Input: part model. Units: mm. Frame: model coordinates. A direction names the side the tool comes from. Coordinates: 2 decimals unless noted, no trailing zeros. Order: outer loops, then holes, each group sorted by start corner. A loop starts at its lowest first (then second) coordinate and runs counter-clockwise, first axis right, second up. Notation, with made-up numbers: (68.25, 48.5) -> (98.25, 48.5) arc R15 ccw to (98.25, 58.5) -> close; hole circle Ø10 at (50.5, -8.75). An arc over 180 degrees is marked (long way). Use CSV: the item, a comma, the result in double quotes. Start each with the question number.
```python
from build123d import *

# Parameters (mm, degrees)
BOSS_EXTRUDE1_DEPTH = 180
CUT_EXTRUDE1_REACH  = 186.932
SKETCH2_R           = 4
CUT_EXTRUDE2_REACH  = 186.932
SKETCH3_R           = 4


with BuildPart() as part:
    # Sketch1 → Boss-Extrude1 (new, symmetric)
    with BuildSketch(Plane.XY):
        Polygon((0, 0), (-30, 0), (-30, -2), (-2, -2), (-2, -30), (0, -30), align=None)
    extrude(amount=BOSS_EXTRUDE1_DEPTH, both=True)

    # Sketch2 → Cut-Extrude1 (cut, up to next)
    with BuildSketch(Plane(origin=(0, 0, 0), x_dir=(1, 0, 0), z_dir=(0, 1, 0)), mode=Mode.PRIVATE) as cut_extrude1_sk1:
        with Locations(Location((-15, 170, 0), (0, 0, 180))):
            Circle(SKETCH2_R)
    cut_extrude1_tool1 = extrude(cut_extrude1_sk1.sketch, amount=-CUT_EXTRUDE1_REACH, mode=Mode.PRIVATE) & part.part
    cut_extrude1 = cut_extrude1_tool1.solids().sort_by_distance((-15, 0, -170))[0]
    add(cut_extrude1, mode=Mode.SUBTRACT)

    # Sketch3 → Cut-Extrude2 (cut, up to next)
    with BuildSketch(Plane(origin=(0, 0, 0), x_dir=(0, 0, -1), z_dir=(1, 0, 0)), mode=Mode.PRIVATE) as cut_extrude2_sk1:
        with Locations(Location((157.5, -15, 0), (0, 0, 90))):
            Circle(SKETCH3_R)
    cut_extrude2_tool1 = extrude(cut_extrude2_sk1.sketch, amount=-CUT_EXTRUDE2_REACH, mode=Mode.PRIVATE) & part.part
    cut_extrude2 = cut_extrude2_tool1.solids().sort_by_distance((0, -15, -157.5))[0]
    add(cut_extrude2, mode=Mode.SUBTRACT)

    # Mirror1: Cut-Extrude1, Cut-Extrude2 across plane
    add(cut_extrude1.mirror(Plane.XY), mode=Mode.SUBTRACT)
    add(cut_extrude2.mirror(Plane.XY), mode=Mode.SUBTRACT)


solid = part.part
```
1. Section A-A on y = -15. Return loops of the section in (x, z).
2. Access query for faces 1 (the face through (-16, -2, 3)), 2 (the face through (-0.986, -15.521, -153.534)). Directions: +Z, -Z, +X, -X, +Y, -Y. A direction counts if a zero-diameter tool reaches every point of the face in a straight line with its end or side. Return the directions, or none.
3. Section B-B on z = 157.5. Return loops of the section in (x, y), then the cut area to 3 significant figures.
4. Material intervals for line 1 along Z through (x, y) = (-15, -1.15); line 2 along Z through (x, y) = (-1.4, -15); line 3 along Y through (x, z) = (-1.35, 157.5), sorted ascending.
5. Section D-D on z = -82.5. Return loops of the section in (x, y), then the cut area to 3 significant figures.
6. Pull-direction query (X, two-part tool) for faces 3 (the face through (-8.4, -1.6, -180)), 4 (the face through (0, -15, 3)), 5 (the face through (-14.479, -0.986, 166.034)); classes: released by +X, released by -X, zero draft, split by the parting line, or undercut.
7. Section C-C on x = -15. Return loops of the section in (y, z), then the cut area to 3 significant figures.
8. Contact query for flat-ended pins moving along their axis: P1, Ø13, axis at x = -15, z = -170, coming from the -Y side; P2, Ø9, axis at y = -15, z = -157.5, coming from the -X side. Output: stop coordinate, or through.
Values follow:
1,outline,"(-2, -180) -> (0, -180) -> (0, -161.5) -> (-2, -161.5) -> close; (-2, -153.5) -> (0, -153.5) -> (0, 153.5) -> (-2, 153.5) -> close; (-2, 161.5) -> (0, 161.5) -> (0, 180) -> (-2, 180) -> close"
2,face 1,"+Z, -Z, -X, -Y"
2,face 2,"+X, -X"
3,outline,"(-30, -2) -> (-2, -2) -> (-2, -11) -> (0, -11) -> (0, 0) -> (-30, 0) -> close; (-2, -30) -> (0, -30) -> (0, -19) -> (-2, -19) -> close"
3,area,"100 mm2"
4,line 1,"z = -180 to -174, -166 to 166, 174 to 180"
4,line 2,"z = -180 to -161.5, -153.5 to 153.5, 161.5 to 180"
4,line 3,"y = -30 to -19, -11 to 0"
5,outline,"(-30, -2) -> (-2, -2) -> (-2, -30) -> (0, -30) -> (0, 0) -> (-30, 0) -> close"
5,area,"116 mm2"
6,face 3,"zero draft"
6,face 4,"released by +X"
6,face 5,"undercut"
7,outline,"(-2, -180) -> (0, -180) -> (0, -174) -> (-2, -174) -> close; (-2, -166) -> (0, -166) -> (0, 166) -> (-2, 166) -> close; (-2, 174) -> (0, 174) -> (0, 180) -> (-2, 180) -> close"
7,area,"688 mm2"
8,P1,"stops at y = -2"
8,P2,"stops at x = -2"
